```python
from build123d import *

# Parameters (mm, degrees)
CROQUIS1_W              = 500
CROQUIS1_H              = 500
SALIENTE_EXTRUIR1_DEPTH = 10
CROQUIS22_W             = 40.5
CROQUIS22_H             = 19.8
CROQUIS22_W_2           = 19.8
CROQUIS22_H_2           = 40.5
CORTAR_EXTRUIR1_DEPTH   = 10
REDONDEO1_R             = 1


with BuildPart() as part:
    # Croquis1 → Saliente-Extruir1 (new body)
    with BuildSketch(Plane(origin=(0, 0, 0), x_dir=(1, 0, 0), z_dir=(0, 1, 0))):
        with Locations((250, 250)):
            Rectangle(CROQUIS1_W, CROQUIS1_H)
    extrude(amount=SALIENTE_EXTRUIR1_DEPTH)

    # Croquis22 → Cortar-Extruir1 (cut)
    with BuildSketch(Plane(origin=(0, 10, 0), x_dir=(1, 0, 0), z_dir=(0, 1, 0))):
        with Locations((50.671999964, 108.122675133)):
            Rectangle(CROQUIS22_W, CROQUIS22_H)
        with Locations((444.021393457, 108.122675133)):
            Rectangle(CROQUIS22_W, CROQUIS22_H)
        with Locations((250, 441.225372138)):
            Rectangle(CROQUIS22_W_2, CROQUIS22_H_2)
    extrude(amount=-CORTAR_EXTRUIR1_DEPTH, mode=Mode.SUBTRACT)

    # Redondeo1
    redondeo1_edges = [part.edges().sort_by_distance(p)[0] for p in [
        (30.421999964, 5, -98.222675133),
        (30.421999964, 5, -118.022675133),
        (70.921999964, 5, -118.022675133),
        (70.921999964, 5, -98.222675133),
        (423.771393457, 5, -98.222675133),
        (423.771393457, 5, -118.022675133),
        (464.271393457, 5, -118.022675133),
        (464.271393457, 5, -98.222675133),
        (240.1, 5, -461.475372138),
        (259.9, 5, -461.475372138),
        (259.9, 5, -420.975372138),
    ]]
    fillet(redondeo1_edges, radius=REDONDEO1_R)


solid = part.part
```
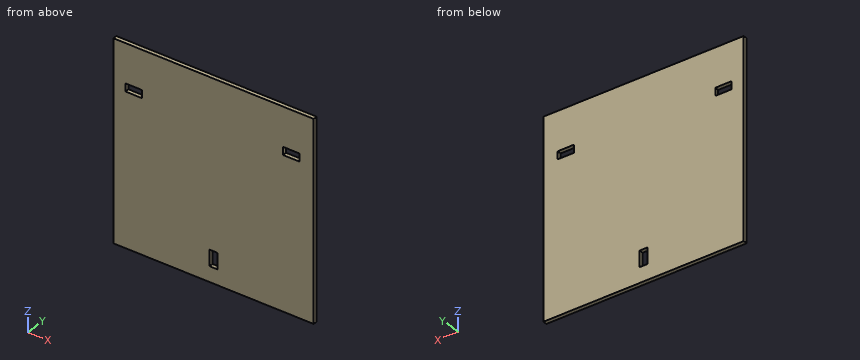
Source: CAD feature listing. Evaluate the final solid. Frame: model axes, mm. Coordinates: 2 decimals unless noted, no trailing zeros. Loops run counter-clockwise (first coordinate to the right, second up) from the corner with the lowest first, then second, coordinate; pieces in that order, holes last. Notation, with made-up numbers: M 60.25,87 L 66.25,87 A15 ccw 66.25,112 Z; hole C 4,83.25 d8. An arc over 180 degrees is marked long. Use CSV: the item, a comma, the result in double quotes.
(1) Line query: line 1 (Z direction, x = 256, y = 8.75); line 2 (Z direction, x = 429, y = 7). Output: solid intervals per line, ascending. Write a range as [from, to].
Answers follow:
line 1,"[-500, -461.48], [-420.98, 0]"
line 2,"[-500, -118.02], [-98.22, 0]"
(2) Cut plane A-A on z = -428. Return loops of the section in (x, y), and give its area (3 significant figures).
Answers follow:
outline,"M 0,0 L 240.1,0 L 240.1,10 L 0,10 Z; M 259.9,0 L 500,0 L 500,10 L 259.9,10 Z"
area,"4,800 mm²"
(3) Contact query for a flat-ended pin moving along its axis: pin 1 (3 mm diameter, centred on x = 314, z = -183.5, fed in from -Y). Output: stop coordinate, or through.
Answers follow:
pin 1,"y = 0"
(4) Cut plane C-C on z = -109. Return loops of the section in (x, y), and give its area (3 significant figures).
Answers follow:
outline,"M 0,0 L 30.42,0 L 30.42,10 L 0,10 Z; M 70.92,0 L 423.77,0 L 423.77,10 L 70.92,10 Z; M 464.27,0 L 500,0 L 500,10 L 464.27,10 Z"
area,"4,190 mm²"
(5) Cut plane B-B on x = 442. Return loops of the section in (y, z).
Answers follow:
outline,"M 0,-500 L 10,-500 L 10,-118.02 L 0,-118.02 Z; M 0,-98.22 L 10,-98.22 L 10,0 L 0,0 Z"
